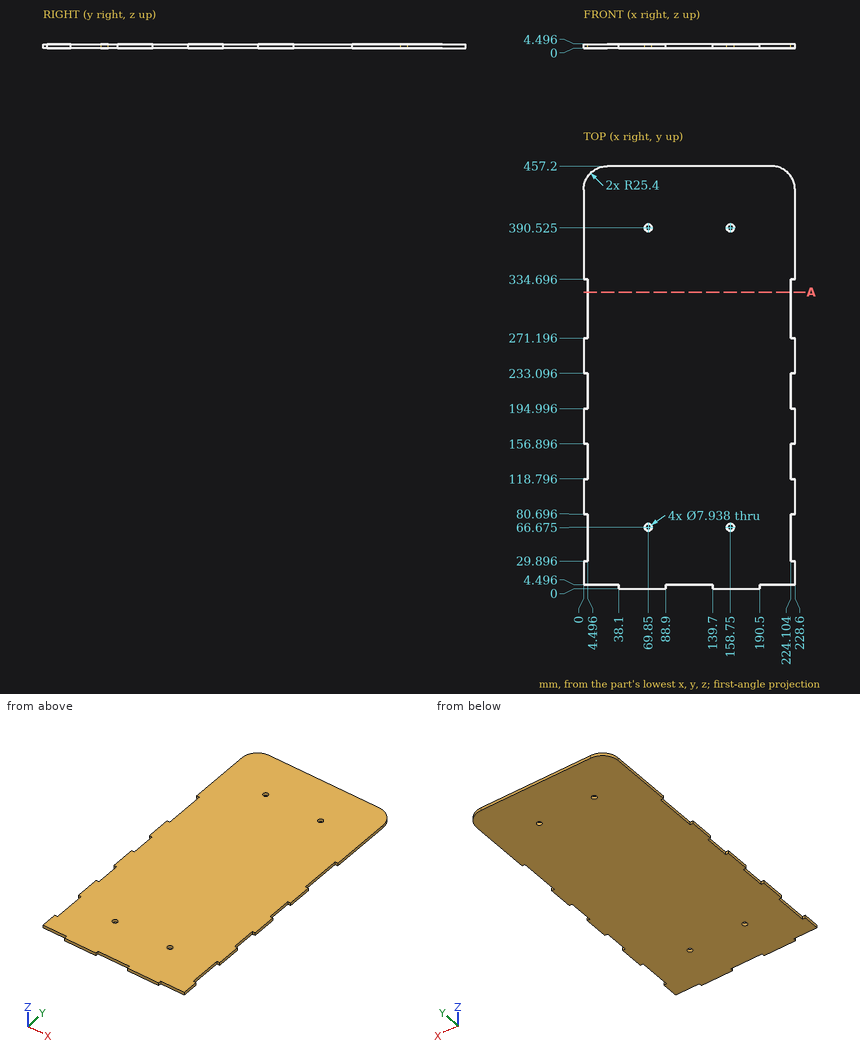
Geometry check sheet. Reference: drawing and pictorial views, mm from the part's lowest x, y, z. Round coordinates to 2 decimals unless told otherwise and drop trailing zeros. Order: outer loops, then holes, each group sorted by start corner. A loop starts at its lowest first (then second) coordinate and runs counter-clockwise, first axis right, second up. Notation, with made-up numbers: M -1,14 L 3,14 A14 ccw 3,35 Z; hole C 7,4.25 d4. An arc over 180 degrees is marked long. Write item = value, one per line.
Q1. Scan lines: line 1 (Y direction, x = 158.75, z = 2.95); line 2 (Y direction, x = 156, z = 2.55) (1 decimal); line 3 (X direction, y = 310, z = 2.4) (1 decimal). Record each from-to range of solid material in increasing order.
Answer block:
line_1 = 0 to 62.71, 70.64 to 386.56, 394.49 to 457.2
line_2 = 0 to 63.8, 69.5 to 387.7, 393.4 to 457.2
line_3 = 4.5 to 224.1
Q2. Section check A-A (y = 321). Enter the section's corners in (x, z) (1 decimal).
Answer block:
outline = M 4.5,0 L 224.1,0 L 224.1,4.5 L 4.5,4.5 Z
Q3. Depth check by flat-ended pin: pin 1 Ø1.3 at (x, z) = (225.5, 1.5) entering from -Y; pin 2 Ø2 at (y, z) = (131.5, 2) entering from -X; pin 3 Ø5 at (x, y) = (158.75, 66.675) entering from +Z; pin 4 Ø1.3 at (x, z) = (225, 2) entering from +Y (1 decimal). Enter the tip coordinate at first touch or a pass-through.
Answer block:
pin_1 = 4.5
pin_2 = 4.5
pin_3 = through
pin_4 = 445.9
